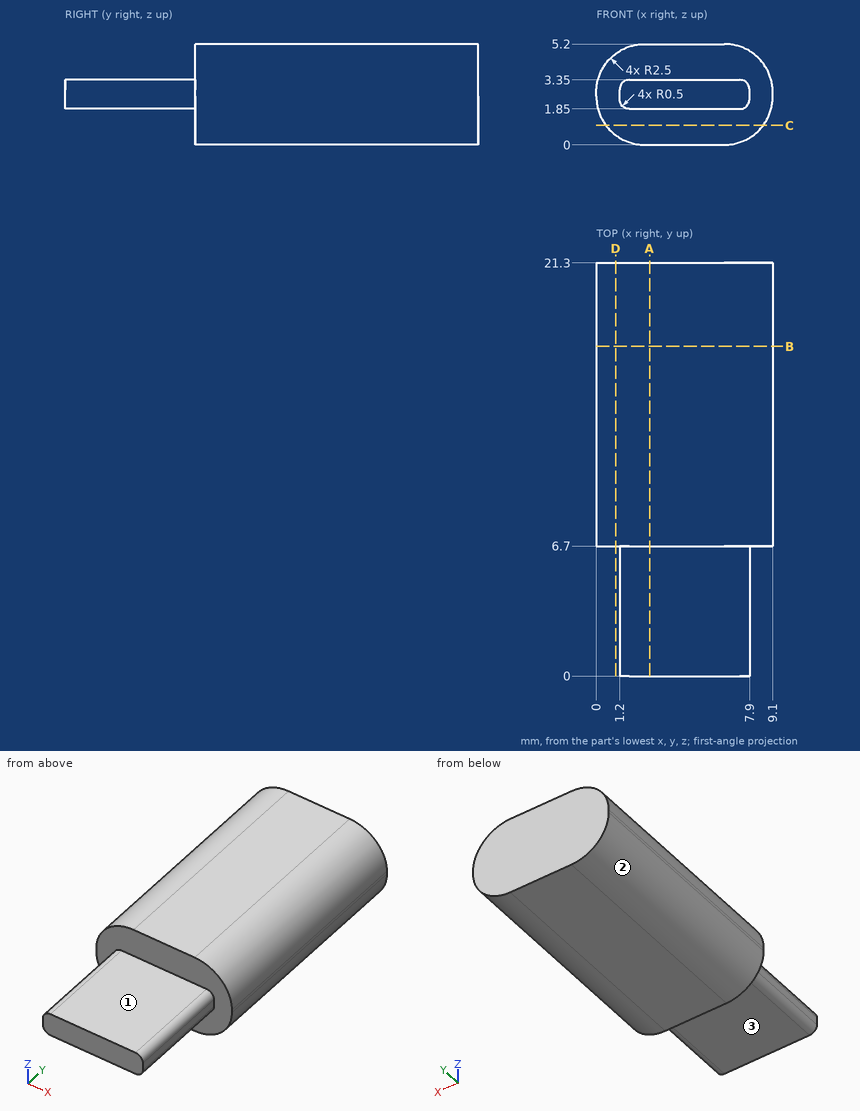
Design review of the part shown in the three views and the two pictorial views. Dimensions are in mm from the part's minimum x, y and z. A direction names the side the tool comes from. Coordinates: 2 decimals unless noted, no trailing zeros. Order: outer loops, then holes, each group sorted by start corner. A loop starts at its lowest first (then second) coordinate and runs counter-clockwise, first axis right, second up.
Item 1: For pin 1 Ø1 at (y, z) = (6.5, 3.5) entering from +X; pin 2 Ø3 at (x, y) = (5.5, 3) entering from +Z; pin 3 Ø3 at (y, z) = (18, 1) entering from -X; pin 4 Ø4 at (x, y) = (7.5, 4) entering from -Z, all flat-tipped, find the tip position at first contact; note any pin that passes through.
Item 2: For line 1 (Y direction, x = 4.75, z = 4.7); line 2 (X direction, y = 20, z = 2.4); line 3 (Z direction, x = 6.25, y = 4.5), list the stretches that pass through material, from the lowest coordinate up.
Item 3: Take a section at C-C, the plane z = 1. Write out the cut boundary in (x, y).
Item 4: For the marked faces 1, 2 and 3, list the 3-axis set-ups (+Z, -Z, +X, -X, +Y, -Y) from which the entire face can be reached by the end or side of a thin tool; tool diameter is ignored.
Item 5: Take a section at B-B, the plane y = 17. Write out the cut boundary in (x, z).
Item 6: Take a section at A-A, the plane x = 2.75. Write out the cut boundary in (y, z).
Item 7: Take a section at D-D, the plane x = 1. Write out the cut boundary in (y, z).
The answers:
1. pin 1: stops at x = 9.08
1. pin 2: stops at z = 3.35
1. pin 3: stops at x = 0
1. pin 4: stops at z = 1.85
2. line 1: y = 6.7 to 21.3
2. line 2: x = 0 to 9.1
2. line 3: z = 1.85 to 3.35
3. outline: (0.5, 6.7) - (8.6, 6.7) - (8.6, 21.3) - (0.5, 21.3) - close
4. face 1: +Z, +X, -X, -Y
4. face 2: -Z, -X, +Y, -Y
4. face 3: -Z, +X, -X, -Y
5. outline: (0, 2.5) arc R2.5 ccw to (2.5, 0) - (6.6, 0) arc R2.5 ccw to (9.1, 2.5) - (9.1, 2.7) arc R2.5 ccw to (6.6, 5.2) - (2.5, 5.2) arc R2.5 ccw to (0, 2.7) - close
6. outline: (0, 1.85) - (6.7, 1.85) - (6.7, 0) - (21.3, 0) - (21.3, 5.2) - (6.7, 5.2) - (6.7, 3.35) - (0, 3.35) - close
7. outline: (6.7, 0.5) - (21.3, 0.5) - (21.3, 4.7) - (6.7, 4.7) - close
